from build123d import *

# Parameters (mm, degrees)
BOX003_W     = 8
BOX003_H     = 180
BOX003_DEPTH = 1.5
BOX004_W     = 8
BOX004_H     = 1.5
BOX004_DEPTH = 52
BOX005_W     = 8
BOX005_H     = 1.5
BOX005_DEPTH = 52
BOX002_W     = 12
BOX002_H     = 180
BOX002_DEPTH = 52
BOX_W        = 160
BOX_H        = 180
BOX_DEPTH    = 50
BOX001_W     = 92
BOX001_H     = 184
BOX001_DEPTH = 54
FILLET_R     = 1.5


with BuildPart() as cube003:
    # Box003 → Box003 (new body)
    with BuildSketch(Plane.XY.offset(48.5)):
        with Locations((4, 90)):
            Rectangle(BOX003_W, BOX003_H)
    extrude(amount=BOX003_DEPTH)


with BuildPart() as cube004:
    # Box004 → Box004 (new body)
    with BuildSketch(Plane.XY.offset(-2)):
        with Locations((4, 0.75)):
            Rectangle(BOX004_W, BOX004_H)
    extrude(amount=BOX004_DEPTH)


with BuildPart() as cube005:
    # Box005 → Box005 (new body)
    with BuildSketch(Plane(origin=(0, 178.5, -2), x_dir=(1, 0, 0), z_dir=(0, 0, 1))):
        with Locations((4, 0.75)):
            Rectangle(BOX005_W, BOX005_H)
    extrude(amount=BOX005_DEPTH)


with BuildPart() as cube002:
    # Box002 → Box002 (new body)
    with BuildSketch(Plane.XY.offset(-20)):
        with Locations((6, 90)):
            Rectangle(BOX002_W, BOX002_H)
    extrude(amount=BOX002_DEPTH)


with BuildPart() as cube:
    # Box → Box (new body)
    with BuildSketch(Plane.XY):
        with Locations((80, 90)):
            Rectangle(BOX_W, BOX_H)
    extrude(amount=BOX_DEPTH)


with BuildPart() as draft:
    # Box001 → Box001 (new body)
    with BuildSketch(Plane(origin=(0, -2, -2), x_dir=(1, 0, 0), z_dir=(0, 0, 1))):
        with Locations((46, 92)):
            Rectangle(BOX001_W, BOX001_H)
    extrude(amount=BOX001_DEPTH)

    # Cut: cut Cube
    add(cube.part, mode=Mode.SUBTRACT)

    # Cut001: cut Cube002
    add(cube002.part, mode=Mode.SUBTRACT)

    # Fusion: union Cube003, Cube004, Cube005
    add(cube003.part)
    add(cube004.part)
    add(cube005.part)

    # Fillet
    fillet_edges = [draft.edges().sort_by_distance(p)[0] for p in [
        (0, 90, 52),
        (0, 182, 25),
        (0, -2, 25),
        (46, 182, 52),
    ]]
    fillet(fillet_edges, radius=FILLET_R)


solid = draft.part
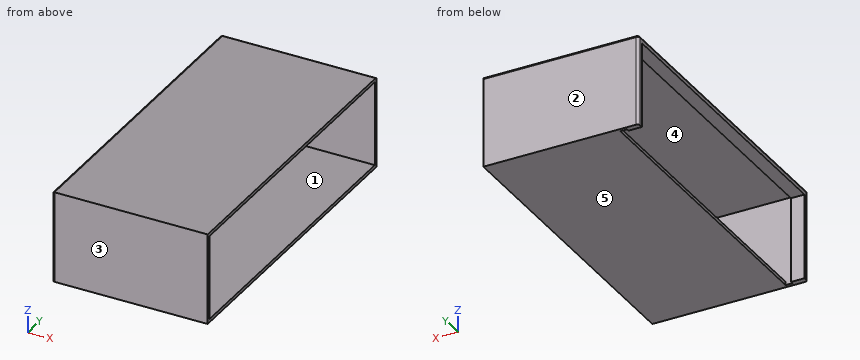
Geometry: final body of the model. Coordinates: model frame, mm. Face numbers are marked on the shaded views. A direction names the side the tool comes from. Give positions to 0.01 mm unless a question says otherwise; leave off trailing zeros. Loops run counter-clockwise (first coordinate to the right, second up) from the corner with the lowest first, then second, coordinate; pieces in that order, holes last. Notation, with made-up numbers: (82.25, -26.5) - (106.25, -26.5) arc R21 cw to (106.25, -2.5) - close; hole circle Ø7 at (47.25, 81). An arc over 180 degrees is marked (long way). One line per question, with ' | ' between items. Start each with the question number.
(1) Section query B-B on y = 110. Return loops of the section in (x, z), then the cut area to 3 significant figures.
(2) Contact query for flat-ended pins moving along their axis: pin 1 (2.5 mm diameter, centred on x = 3, y = 63.5, fed in from -Z); pin 2 (0.6 mm diameter, centred on y = 46.5, z = -0.5, fed in from -X). Output: stop coordinate, or through.
(3) Ray query, line 1 (Y direction, x = 82.5, z = 10); line 2 (Y direction, x = 5.5, z = 6.5); line 3 (Z direction, x = 53, y = 99). Return the intervals inside material, ascending. Write a range as from..to.
(4) Section query C-C on z = 26. Return loops of the section in (x, y), then the cut area to 3 significant figures.
(5) Pull-direction query (Y, two-part tool) for the marked faces 1, 2 and 3; classes: released by +Y, released by -Y, zero draft, split by the parting line, or undercut.
(6) Section query A-A on x = 31. Return loops of the section in (y, z).
(7) Reachability of the marked faces 4 and 5 from +Z, -Z, +X, -X, +Y, -Y: full face, straight path, thin tool, end or side. Return the list, or none.
The answers:
1) outline: (0, 48.5) - (8, 48.5) - (8, 50) - (92, 50) - (92, 52) - (1.5, 52) arc R1.5 ccw to (0, 50.5) - close; (12, -2) - (92, -2) - (92, 0) - (12, 0) - close | area: 356 mm2
2) pin 1: z = 48.5 | pin 2: x = 12
3) line 1: -2..0, 180..182 | line 2: -2..1.5, 178.5..182 | line 3: -2..0, 50..52
4) outline: (0, -0.5) arc R1.5 ccw to (1.5, -2) - (92, -2) - (92, 0) - (8, 0) - (8, 1.5) - (0, 1.5) - close; (0, 178.5) - (8, 178.5) - (8, 180) - (92, 180) - (92, 182) - (1.5, 182) arc R1.5 ccw to (0, 180.5) - close | area: 391 mm2
5) face 1: undercut | face 2: released by +Y | face 3: released by -Y
6) outline: (-2, -2) - (182, -2) - (182, 50.5) arc R1.5 ccw to (180.5, 52) - (-2, 52) - close; hole (0, 0) - (180, 0) - (180, 50) - (0, 50) - close
7) face 4: +X | face 5: -Z, +X, -X, +Y, -Y
